from build123d import *

# Parameters (mm, degrees)
SKETCH_1_R                   = 50
EXTRUDE_1_DEPTH              = 5
HOLE_WIZARD_M2_1_D           = 2.4
HOLE_WIZARD_M2_1_CBORE_D     = 4.2
HOLE_WIZARD_M2_1_CBORE_DEPTH = 1.45
HOLE_WIZARD_M3_2_D           = 3.4
HOLE_WIZARD_M3_2_CBORE_D     = 6.05
HOLE_WIZARD_M3_2_CBORE_DEPTH = 2.2
PATTERN_CIRCULAR_1_COUNT     = 8
SKETCH_6_R                   = 8.5
CUT_EXTRUDE_1_DEPTH          = 71.887234394
SKETCH_7_R                   = 5.4875
CUT_EXTRUDE_2_DEPTH          = 71.887234394
FILLET_1_R                   = 1.5
HOLE_WIZARD_M3_3_D           = 3.4
HOLE_WIZARD_M3_3_CBORE_D     = 6.05
HOLE_WIZARD_M3_3_CBORE_DEPTH = 2.2
SKETCH_12_W                  = 5
SKETCH_12_H                  = 2
CUT_EXTRUDE_4_DEPTH          = 71.887234394
SKETCH_14_W                  = 2
SKETCH_14_H                  = 5
EXTRUDE_2_DEPTH              = 3
FILLET_2_R                   = 1
FILLET_2_OF_MIRROR_2_R       = 1
CUT_EXTRUDE_5_DEPTH          = 72.161787499


with BuildPart() as part:
    # ｽｹｯﾁ1 → ﾎﾞｽ - 押し出し1 (new body)
    with BuildSketch(Plane.XY):
        Circle(SKETCH_1_R)
    extrude(amount=EXTRUDE_1_DEPTH)

    # M2 丸平ねじ用座ぐり穴1 (through all)
    with Locations(Plane.XY.offset(5)):
        with Locations((-10.5, 0), (-10.5, -21)):
            hole_wizard_m2_1 = CounterBoreHole(HOLE_WIZARD_M2_1_D / 2, HOLE_WIZARD_M2_1_CBORE_D / 2, HOLE_WIZARD_M2_1_CBORE_DEPTH)

    # ﾐﾗｰ1: M2 丸平ねじ用座ぐり穴1 across plane
    add(hole_wizard_m2_1.mirror(Plane(origin=(0, 0, 0), x_dir=(0, 0, 1), z_dir=(1, 0, 0))), mode=Mode.SUBTRACT)

    # M3 丸平ねじ用座ぐり穴2 (through all)
    with Locations(Plane.XY.offset(5)):
        with Locations((46, 0)):
            hole_wizard_m3_2 = CounterBoreHole(HOLE_WIZARD_M3_2_D / 2, HOLE_WIZARD_M3_2_CBORE_D / 2, HOLE_WIZARD_M3_2_CBORE_DEPTH)

    # 円形ﾊﾟﾀｰﾝ1: M3 丸平ねじ用座ぐり穴2 ×8 about axis
    pattern_circular_1_axis = Axis((0, 0, 0), (0, 0, 1))
    for i in range(1, PATTERN_CIRCULAR_1_COUNT):
        add(hole_wizard_m3_2.rotate(pattern_circular_1_axis, i * 360 / PATTERN_CIRCULAR_1_COUNT), mode=Mode.SUBTRACT)

    # ｽｹｯﾁ6 → ｶｯﾄ - 押し出し1 (cut, through all)
    with BuildSketch(Plane.XY.offset(5)):
        Circle(SKETCH_6_R)
    extrude(amount=-CUT_EXTRUDE_1_DEPTH, mode=Mode.SUBTRACT)

    # ｽｹｯﾁ7 → ｶｯﾄ - 押し出し2 (cut, through all)
    with BuildSketch(Plane.XY.offset(5)):
        with Locations((0, -35.4875)):
            Circle(SKETCH_7_R)
    extrude(amount=-CUT_EXTRUDE_2_DEPTH, mode=Mode.SUBTRACT)

    # ﾌｨﾚｯﾄ1
    fillet_1_edges = [part.edges().sort_by_distance(p)[0] for p in [
        (-5.4875, -35.4875, 0),
        (-5.4875, -35.4875, 5),
    ]]
    fillet(fillet_1_edges, radius=FILLET_1_R)

    # M3 丸平ねじ用座ぐり穴3 (through all)
    with Locations(Plane.XY.offset(5)):
        with Locations((22, -2), (22, -12)):
            CounterBoreHole(HOLE_WIZARD_M3_3_D / 2, HOLE_WIZARD_M3_3_CBORE_D / 2, HOLE_WIZARD_M3_3_CBORE_DEPTH)

    # ｽｹｯﾁ12 → ｶｯﾄ - 押し出し4 (cut, through all)
    with BuildSketch(Plane(origin=(0, 0, 0), x_dir=(-1, 0, 0), z_dir=(0, 0, -1))):
        with Locations((16.5, 35)):
            Rectangle(SKETCH_12_W, SKETCH_12_H)
        with Locations((16.5, 10.5)):
            Rectangle(SKETCH_12_W, SKETCH_12_H)
    cut_extrude_4 = extrude(amount=-CUT_EXTRUDE_4_DEPTH, mode=Mode.SUBTRACT)

    # ｽｹｯﾁ14 → ﾎﾞｽ - 押し出し2 (add)
    with BuildSketch(Plane(origin=(0, 0, 0), x_dir=(-1, 0, 0), z_dir=(0, 0, -1))):
        with Locations((25, 29.5)):
            Rectangle(SKETCH_14_W, SKETCH_14_H)
        with Locations((25, 16)):
            Rectangle(SKETCH_14_W, SKETCH_14_H)
    extrude_2 = extrude(amount=EXTRUDE_2_DEPTH)

    # ﾌｨﾚｯﾄ2
    fillet_2_edges = [part.edges().sort_by_distance(p)[0] for p in [
        (-26, 29.5, 0),
        (-26, 16, 0),
    ]]
    fillet(fillet_2_edges, radius=FILLET_2_R)

    # ﾐﾗｰ2: ｶｯﾄ - 押し出し4, ﾎﾞｽ - 押し出し2 across plane
    add(cut_extrude_4.mirror(Plane(origin=(0, 0, 0), x_dir=(0, 0, 1), z_dir=(1, 0, 0))), mode=Mode.SUBTRACT)
    add(extrude_2.mirror(Plane(origin=(0, 0, 0), x_dir=(0, 0, 1), z_dir=(1, 0, 0))))

    # ﾌｨﾚｯﾄ2 of ﾐﾗｰ2
    fillet_2_of_mirror_2_edges = [part.edges().sort_by_distance(p)[0] for p in [
        (26, 29.5, 0),
        (26, 16, 0),
    ]]
    fillet(fillet_2_of_mirror_2_edges, radius=FILLET_2_OF_MIRROR_2_R)

    # ｽｹｯﾁ15 → ｶｯﾄ - 押し出し5 (cut, through all)
    with BuildSketch(Plane.XY.offset(5)):
        with BuildLine():
            Line((-29, -5.5), (-29, -11.5))
            ThreePointArc((-29, -11.5), (-34, -16.5), (-39, -11.5))
            Line((-39, -11.5), (-39, -5.5))
            ThreePointArc((-39, -5.5), (-34, -0.5), (-29, -5.5))
        make_face()
    extrude(amount=-CUT_EXTRUDE_5_DEPTH, mode=Mode.SUBTRACT)


solid = part.part
Input: part model. Units: mm. Frame: model coordinates. A direction names the side the tool comes from. Give positions to 0.01 mm unless a question says otherwise; leave off trailing zeros. Order: outer loops, then holes, each group sorted by start corner. A loop starts at its lowest first (then second) coordinate and runs counter-clockwise, first axis right, second up. Notation, with made-up numbers: (-23.75, 82) - (-8.75, 82) arc R17 cw to (-8.75, 110) - close; hole circle Ø1 at (-12.5, -14). An arc over 180 degrees is marked (long way). Answer as a JSON object with one key per item and string values. Group by question number.
Q1. Cut plane B-B, the plane y = 46. Output: boundary loops of the cut face in (x, z) (3 decimals).
Q2. Cut plane A-A, the plane x = 22. Output: boundary loops of the cut face in (y, z) (3 decimals).
Q3. Line query: probe 1 along Y at (x, z) = (22, 2.25); probe 2 along X at (y, z) = (31, 3); probe 3 along Y at (x, z) = (15.5, 2.5). Output: solid intervals per line, ascending.
Q4. Mould query, pull axis Y, two halves, no side actions, for faces 1 (the face through (-32.5, 34.4, 2.8)), 2 (the face through (24, 16, -1)), 3 (the face through (-25, 13.5, -1)). Classes: pulls with the +Y half, pulls with the -Y half, needs draft (parallel to the pull), parting line crosses it, or undercut.
Q5. Cut plane D-D, the plane x = 10.5. Output: boundary loops of the cut face in (y, z).
Q6. First-contact query: pin 1 Ø3.5 at (x, y) = (22, -12) entering from +Z; pin 2 Ø3.5 at (x, z) = (-25.5, -1.5) entering from -Y; pin 3 Ø1.6 at (y, z) = (10, 2.5) entering from -X. Flat tips, straight axial feed; report the tip coordinate or a pass-through.
Q7. Set-up query: faces 4 (the face through (-16, 11.5, 2)), 5 (the face through (-25, 18.5, -1)), 6 (the face through (18.978, -11.867, 3.915)). Return all of +Z, -Z, +X, -X, +Y, -Y with unobstructed straight access to the full face (end or side cutting, diameter ignored); none if empty.
Results:
{
 "1": {"outline": "(-19.596, 0) - (-1.7, 0) - (-1.7, 2.8) - (-3.025, 2.8) - (-3.025, 5) - (-19.596, 5) - close; (1.7, 0) - (19.596, 0) - (19.596, 5) - (3.025, 5) - (3.025, 2.8) - (1.7, 2.8) - close"},
 "2": {"outline": "(-44.9, 0) - (-13.7, 0) - (-13.7, 2.8) - (-15.025, 2.8) - (-15.025, 5) - (-44.9, 5) - close; (-10.3, 0) - (-3.7, 0) - (-3.7, 2.8) - (-5.025, 2.8) - (-5.025, 5) - (-8.975, 5) - (-8.975, 2.8) - (-10.3, 2.8) - close; (-0.3, 0) - (44.9, 0) - (44.9, 5) - (1.025, 5) - (1.025, 2.8) - (-0.3, 2.8) - close"},
 "3": {"probe 1": "-44.9 to -13.7, -10.3 to -3.7, -0.3 to 44.9", "probe 2": "-39.23 to -35.14, -29.92 to 29.92, 35.14 to 39.23", "probe 3": "-47.54 to 9.5, 11.5 to 34, 36 to 47.54"},
 "4": {"face 1": "undercut", "face 2": "needs draft", "face 3": "pulls with the -Y half"},
 "5": {"outline": "(-48.89, 0) - (-22.2, 0) - (-22.2, 3.55) - (-23.1, 3.55) - (-23.1, 5) - (-48.89, 5) - close; (-19.8, 0) - (-1.2, 0) - (-1.2, 3.55) - (-2.1, 3.55) - (-2.1, 5) - (-18.9, 5) - (-18.9, 3.55) - (-19.8, 3.55) - close; (1.2, 0) - (48.89, 0) - (48.89, 5) - (2.1, 5) - (2.1, 3.55) - (1.2, 3.55) - close"},
 "6": {"pin 1": "z = 2.8", "pin 2": "y = -43.53", "pin 3": "x = -49.15"},
 "7": {"face 4": "+Z, -Z", "face 5": "-Z, +X, -X", "face 6": "+Z"}
}
